Check sheet for the modelled part. Datum: model origin and axes. Units: mm. Face numbers are marked on the shaded views. Round coordinates to 2 decimals unless told otherwise and drop trailing zeros. Order: outer loops, then holes, each group sorted by start corner. A loop starts at its lowest first (then second) coordinate and runs counter-clockwise, first axis right, second up. Notation, with made-up numbers: (79.5, -13) -> (126.5, -13) arc R9 cw to (126.5, 3) -> close; hole circle Ø3 at (84, -18.75). An arc over 180 degrees is marked (long way). Answer in a Markdown table with one row per item.
```python
from build123d import *

# Parameters (mm, degrees)
SKETCH001_R        = 2.15
POCKET_DEPTH       = 5
POLARPATTERN_COUNT = 6
CHAMFER_SIZE       = 2


with BuildPart() as part:
    # Sketch → Revolution (revolve)
    with BuildSketch(Plane.XY):
        Polygon((-8.5, 52), (-5.5, 52), (-5.5, 65.5), (-2.5, 65.5), (-2.5, 52), (0, 52), (0, 49), (-8.5, 49), align=None)
    revolve(axis=Axis((0, 0, 0), (1, 0, 0)))

    # Sketch001 → Pocket (cut)
    with BuildSketch(Plane(origin=(-5.5, 0, 0), x_dir=(0, -1, 0), z_dir=(-1, 0, 0))):
        with Locations((0, 59.5)):
            Circle(SKETCH001_R)
    pocket = extrude(amount=-POCKET_DEPTH, mode=Mode.SUBTRACT)

    # PolarPattern: Pocket ×6 about axis
    polarpattern_axis = Axis((-5.5, 0, 0), (-1, 0, 0))
    for i in range(1, POLARPATTERN_COUNT):
        add(pocket.rotate(polarpattern_axis, i * 360 / POLARPATTERN_COUNT), mode=Mode.SUBTRACT)

    # Chamfer
    chamfer_edges = [part.edges().sort_by_distance(p)[0] for p in [
        (-5.5, 2.15, 59.5),
        (-5.5, 52.603512, 27.888045),
        (-5.5, 50.453512, -31.611955),
        (-5.5, -2.15, -59.5),
        (-5.5, -52.603512, -27.888045),
        (-5.5, -50.453512, 31.611955),
    ]]
    chamfer(chamfer_edges, length=CHAMFER_SIZE)


solid = part.part
```
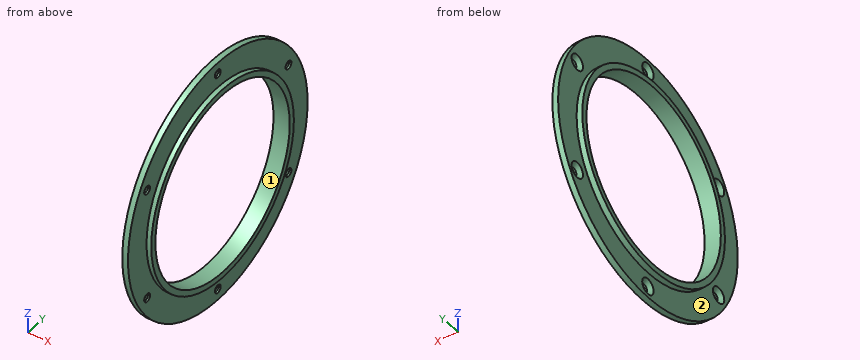
(1) Draft check along Z on the marked faces 1 and 2. Enter one of: pulls with the +Z half, pulls with the -Z half, needs draft (parallel to the pull), parting line crosses it, or undercut.
Solutions:
| item | result |
|---|---|
| face 1 | undercut |
| face 2 | needs draft |
(2) Section check D-D on y = -14. Record the boundary of the cut face in (x, z).
Solutions:
| item | result |
|---|---|
| outline | (-8.5, -50.08) -> (-5.5, -50.08) -> (-5.5, -63.99) -> (-2.5, -63.99) -> (-2.5, -50.08) -> (0, -50.08) -> (0, -46.96) -> (-8.5, -46.96) -> close; (-8.5, 46.96) -> (0, 46.96) -> (0, 50.08) -> (-2.5, 50.08) -> (-2.5, 63.99) -> (-5.5, 63.99) -> (-5.5, 50.08) -> (-8.5, 50.08) -> close |
(3) Section check A-A on z = 0. Record the boundary of the cut face in (x, y), plus the area to 3 significant figures.
Solutions:
| item | result |
|---|---|
| outline | (-8.5, -52) -> (-5.5, -52) -> (-5.5, -65.5) -> (-2.5, -65.5) -> (-2.5, -52) -> (0, -52) -> (0, -49) -> (-8.5, -49) -> close; (-8.5, 49) -> (0, 49) -> (0, 52) -> (-2.5, 52) -> (-2.5, 65.5) -> (-5.5, 65.5) -> (-5.5, 52) -> (-8.5, 52) -> close |
| area | 132 mm^2 |
(4) Depth check by flat-ended pin: pin 1 Ø1 at (x, z) = (-6.5, -18.5) entering from +Y; pin 2 Ø5.5 at (y, z) = (51.53, -29.75) entering from +X; pin 3 Ø1.5 at (x, y) = (-2, -9) entering from +Z; pin 4 Ø3.5 at (y, z) = (-51.53, 29.75) entering from -X. Enter the tip coordinate at first touch or a pass-through.
Solutions:
| item | result |
|---|---|
| pin 1 | y = 48.79 |
| pin 2 | x = -2.5 |
| pin 3 | z = 64.95 |
| pin 4 | through |
(5) Section check C-C on z = 29.75. Record the boundary of the cut face in (x, y), plus the area to 3 significant figures.
Solutions:
| item | result |
|---|---|
| outline | (-8.5, -42.65) -> (-5.5, -42.65) -> (-5.5, -47.38) -> (-3.5, -49.38) -> (-2.5, -49.38) -> (-2.5, -42.65) -> (0, -42.65) -> (0, -38.94) -> (-8.5, -38.94) -> close; (-8.5, 38.94) -> (0, 38.94) -> (0, 42.65) -> (-2.5, 42.65) -> (-2.5, 49.38) -> (-3.5, 49.38) -> (-5.5, 47.38) -> (-5.5, 42.65) -> (-8.5, 42.65) -> close; (-5.5, -58.35) -> (-2.5, -58.35) -> (-2.5, -53.68) -> (-3.5, -53.68) -> (-5.5, -55.68) -> close; (-5.5, 55.68) -> (-3.5, 53.68) -> (-2.5, 53.68) -> (-2.5, 58.35) -> (-5.5, 58.35) -> close |
| area | 124 mm^2 |
(6) Scan lines: probe 1 along Z at (x, y) = (-6.75, -32); probe 2 along X at (y, z) = (-43.5, -39); probe 3 along Z at (x, y) = (-7.75, 30). Record each from-to range of solid material in increasing order. Write a range as from..to.
Solutions:
| item | result |
|---|---|
| probe 1 | -40.99..-37.11, 37.11..40.99 |
| probe 2 | -5.5..-2.5 |
| probe 3 | -42.47..-38.74, 38.74..42.47 |
(7) Section check B-B on y = 0. Record the boundary of the cut face in (x, z), plus the area to 3 significant figures.
Solutions:
| item | result |
|---|---|
| outline | (-8.5, -52) -> (-5.5, -52) -> (-5.5, -55.35) -> (-3.5, -57.35) -> (-2.5, -57.35) -> (-2.5, -52) -> (0, -52) -> (0, -49) -> (-8.5, -49) -> close; (-8.5, 49) -> (0, 49) -> (0, 52) -> (-2.5, 52) -> (-2.5, 57.35) -> (-3.5, 57.35) -> (-5.5, 55.35) -> (-5.5, 52) -> (-8.5, 52) -> close; (-5.5, -65.5) -> (-2.5, -65.5) -> (-2.5, -61.65) -> (-3.5, -61.65) -> (-5.5, -63.65) -> close; (-5.5, 63.65) -> (-3.5, 61.65) -> (-2.5, 61.65) -> (-2.5, 65.5) -> (-5.5, 65.5) -> close |
| area | 98.2 mm^2 |
